For this review, use the dimensioned drawing (mm, ordinates from the lowest corner) and the shaded views. A direction names the side the tool comes from. Round coordinates to 2 decimals unless told otherwise and drop trailing zeros. Loops run counter-clockwise (first coordinate to the right, second up) from the corner with the lowest first, then second, coordinate; pieces in that order, holes last.
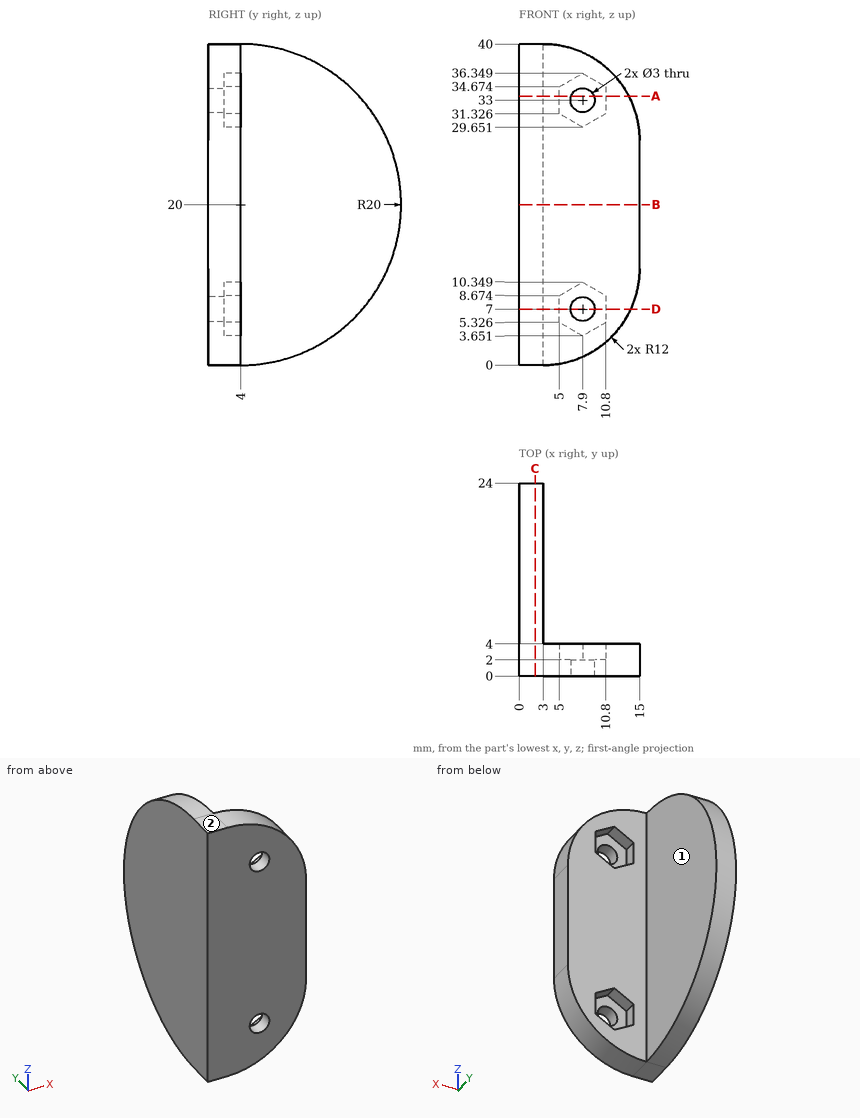
(1) Add section A-A (z = 33.5). Give the boundary of the cut face in (x, y) (1 decimal).
(2) For the marked faces 1 and 2, list the 3-axis set-ups (+Z, -Z, +X, -X, +Y, -Y) from which the entire face can be reached by the end or side of a thin tool; tool diameter is ignored.
(3) Add section D-D (z = 7). Give the boundary of the cut face in (x, y).
(4) Add section C-C (x = 2). Give the boundary of the cut face in (y, z), plus the area to 3 significant figures.
(5) Add section B-B (z = 20). Give the boundary of the cut face in (x, y), plus the area to 3 significant figures.
(6) For L1, parallel to Y at x = 6, z = 22; L2, parallel to X at y = 16.5, z = 29; L3, parallel to X at y = 0.9, z = 7, list the stretches that pass through material, from the lowest coordinate up.
(7) Insertion check: pin 1 Ø6 at (x, z) = (4.5, 4.5) entering from -Y; pin 2 Ø6 at (y, z) = (15.5, 21.5) entering from +X; pin 3 Ø4.5 at (x, z) = (7, 34.5) entering from +Y; pin 4 Ø1.5 at (x, z) = (9.5, 6) entering from +Y. Each pin has a flat end and moves straight along its axis. Give the tip position at first contact, or say it passes through.
Outcome:
1. outline: (0, 0) - (6.5, 0) - (6.5, 2) - (5, 2) - (5, 4) - (3, 4) - (3, 18.8) - (0, 18.8) - close; (9.3, 0) - (13.7, 0) - (13.7, 4) - (10.8, 4) - (10.8, 2) - (9.3, 2) - close
2. face 1: +Z, -Z, +X, +Y
2. face 2: +Z, +X, -X, +Y, -Y
3. outline: (0, 0) - (6.4, 0) - (6.4, 2) - (5, 2) - (5, 4) - (3, 4) - (3, 19.2) - (0, 19.2) - close; (9.4, 0) - (13.91, 0) - (13.91, 4) - (10.8, 4) - (10.8, 2) - (9.4, 2) - close
4. outline: (0, 0) - (4, 0) arc R20 ccw to (4, 40) - (0, 40) - close
4. area: 788 mm2
5. outline: (0, 0) - (15, 0) - (15, 4) - (3, 4) - (3, 24) - (0, 24) - close
5. area: 120 mm2
6. L1: y = 0 to 4
6. L2: x = 0 to 3
6. L3: x = 0 to 6.4, 9.4 to 13.91
7. pin 1: stops at y = 0
7. pin 2: stops at x = 3
7. pin 3: stops at y = 4
7. pin 4: stops at y = 2
